For this review, take the finished solid that the model builds, in its own axes (mm). Give positions to 0.01 mm unless a question says otherwise; leave off trailing zeros. Order: outer loops, then holes, each group sorted by start corner. A loop starts at its lowest first (then second) coordinate and runs counter-clockwise, first axis right, second up.
from build123d import *

# Parameters (mm, degrees)
ESQUISSE1_W             = 30
ESQUISSE1_H             = 51
ESQUISSE1_W_2           = 20
ESQUISSE1_H_2           = 41
BOSS_EXTRU_1_DEPTH      = 5
BOSS_EXTRU_3_DEPTH      = 5
BOSS_EXTRU_4_DEPTH      = 8
ESQUISSE5_W             = 30
ESQUISSE5_H             = 5
BOSS_EXTRU_5_DEPTH      = 2.5
ESQUISSE6_W             = 30
ESQUISSE6_H             = 5
BOSS_EXTRU_6_DEPTH      = 2.5
ESQUISSE7_R             = 1.5
ENL_V_MAT_EXTRU_1_DEPTH = 150.584223767
ESQUISSE8_R             = 2.625
ENL_V_MAT_EXTRU_2_DEPTH = 150.584223767
BOSS_EXTRU_8_DEPTH      = 5
BOSS_EXTRU_9_DEPTH      = 31
BOSS_EXTRU_11_DEPTH     = 5
ESQUISSE16_W            = 17
ESQUISSE16_H            = 10
ESQUISSE16_R            = 1.5
BOSS_EXTRU_12_DEPTH     = 5
CHANFREIN3_SIZE         = 0.25
BOSS_EXTRU_13_DEPTH     = 5
BOSS_EXTRU_14_DEPTH     = 5


with BuildPart() as part:
    # Esquisse1 → Boss.-Extru.1 (new body)
    with BuildSketch(Plane.XY):
        Rectangle(ESQUISSE1_W, ESQUISSE1_H)
        Rectangle(ESQUISSE1_W_2, ESQUISSE1_H_2, mode=Mode.SUBTRACT)
    extrude(amount=BOSS_EXTRU_1_DEPTH)

    # Esquisse3 → Boss.-Extru.3 (add)
    with BuildSketch(Plane(origin=(0, 8, 0), x_dir=(1, 0, 0), z_dir=(0, 1, 0))):
        with BuildLine():
            Line((130.711195077, 0), (15, 0))
            Line((15, 0), (15, -5))
            Line((15, -5), (123.166385806, -5))
            ThreePointArc((123.166385806, -5), (125.435495458, -5.705892931), (126.903730879, -7.574429307))
            Line((126.903730879, -7.574429307), (135, -28.8))
            Line((135, -28.8), (145, -28.8))
            Line((145, -28.8), (134.422141223, -2.507057034))
            ThreePointArc((134.422141223, -2.507057034), (132.950416832, -0.685503668), (130.711195077, 0))
        make_face()
        with BuildLine():
            Line((-123.166385806, -5), (-15, -5))
            Line((-15, -5), (-15, 0))
            Line((-15, 0), (-130.711195077, 0))
            ThreePointArc((-130.711195077, 0), (-132.950416832, -0.685503668), (-134.422141223, -2.507057034))
            Line((-134.422141223, -2.507057034), (-145, -28.8))
            Line((-145, -28.8), (-135, -28.8))
            Line((-135, -28.8), (-126.903730879, -7.574429307))
            ThreePointArc((-126.903730879, -7.574429307), (-125.435495458, -5.705892931), (-123.166385806, -5))
        make_face()
    extrude(amount=-BOSS_EXTRU_3_DEPTH)

    # Esquisse4 → Boss.-Extru.4 (add)
    with BuildSketch(Plane(origin=(0, 8, 0), x_dir=(-1, 0, 0), z_dir=(0, 1, 0))):
        Polygon((145, 28.8), (135, 28.8), (133.09280296, 23.8), (142.98846048, 23.8), align=None)
        Polygon((-142.98846048, 23.8), (-145, 28.8), (-135, 28.8), (-133.09280296, 23.8), align=None)
    extrude(amount=BOSS_EXTRU_4_DEPTH)

    # Esquisse5 → Boss.-Extru.5 (add)
    with BuildSketch(Plane(origin=(0, 25.5, 0), x_dir=(1, 0, 0), z_dir=(0, 1, 0))):
        with Locations((0, -2.5)):
            Rectangle(ESQUISSE5_W, ESQUISSE5_H)
    extrude(amount=BOSS_EXTRU_5_DEPTH)

    # Esquisse6 → Boss.-Extru.6 (add)
    with BuildSketch(Plane.XZ.offset(25.5)):
        with Locations((0, 2.5)):
            Rectangle(ESQUISSE6_W, ESQUISSE6_H)
    extrude(amount=BOSS_EXTRU_6_DEPTH)

    # Esquisse7 → Enlèv. mat.-Extru.1 (cut, through all)
    with BuildSketch(Plane(origin=(0, 0, 23.8), x_dir=(-1, 0, 0), z_dir=(0, 0, -1))):
        with Locations((-140, 10)):
            Circle(ESQUISSE7_R)
        with Locations(Location((140, 10, 0), (0, 0, 180))):
            Circle(ESQUISSE7_R)
    extrude(amount=-ENL_V_MAT_EXTRU_1_DEPTH, mode=Mode.SUBTRACT)

    # Esquisse8 → Enlèv. mat.-Extru.2 (cut, through all)
    with BuildSketch(Plane.XY.offset(5)):
        with Locations((-5, 24.925)):
            Circle(ESQUISSE8_R)
        with Locations((5, 24.925)):
            Circle(ESQUISSE8_R)
        with Locations((-5, -25.425)):
            Circle(ESQUISSE8_R)
        with Locations((5, -25.425)):
            Circle(ESQUISSE8_R)
    extrude(amount=-ENL_V_MAT_EXTRU_2_DEPTH, mode=Mode.SUBTRACT)

    # Esquisse12 → Boss.-Extru.8 (add)
    with BuildSketch(Plane(origin=(0, 8, 0), x_dir=(1, 0, 0), z_dir=(0, 1, 0))):
        Polygon((-129.99826692, -15.687214654), (-63.433313414, -5), (-31.892154123, -5), (-132.055900977, -21.081607615), align=None)
        Polygon((132.055900977, -21.081607615), (129.99826692, -15.687214654), (63.433313414, -5), (31.892154123, -5), align=None)
    extrude(amount=-BOSS_EXTRU_8_DEPTH)

    # Esquisse13 → Boss.-Extru.9 (add, through all)
    with BuildSketch(Plane.XZ.offset(-3)):
        with BuildLine():
            Line((-126.684620904, 7), (-136.229687691, 7))
            Line((-136.229687691, 7), (-134.422141223, 2.507057034))
            ThreePointArc((-134.422141223, 2.507057034), (-132.950416832, 0.685503668), (-130.711195077, 0))
            Line((-130.711195077, 0), (-126.684620904, 0))
            Line((-126.684620904, 0), (-126.684620904, 7))
        make_face()
        with BuildLine():
            ThreePointArc((134.422141223, 2.507057034), (132.950416832, 0.685503668), (130.711195077, 0))
            Line((130.711195077, 0), (126.684620904, 0))
            Line((126.684620904, 0), (126.684620904, 7))
            Line((126.684620904, 7), (136.229687691, 7))
            Line((136.229687691, 7), (134.422141223, 2.507057034))
        make_face()
    extrude(amount=BOSS_EXTRU_9_DEPTH)

    # Esquisse15 → Boss.-Extru.11 (add)
    with BuildSketch(Plane(origin=(-114.828371074, 0, -46.196361295), x_dir=(-0.3732357415464263, 0, 0.9277365365405684), z_dir=(-0.9277365365405683, 0, -0.37323574154642625))):
        Polygon((56.042576064, -14.320508076), (66.042576064, 3), (69.506677679, 3), (56.409919429, -19.684250702), align=None)
    boss_extru_11 = extrude(amount=-BOSS_EXTRU_11_DEPTH)

    # Symétrie3: Boss.-Extru.11 across plane
    add(boss_extru_11.mirror(Plane(origin=(0, 0, 0), x_dir=(0, 0, 1), z_dir=(1, 0, 0))))

    # Esquisse16 → Boss.-Extru.12 (add)
    # profile 1 of 2: a face of its own
    with BuildSketch(Plane.XZ.offset(28)):
        with Locations((131.457154298, 3.5)):
            Rectangle(ESQUISSE16_W, ESQUISSE16_H)
        with Locations(Location((124.957154298, 3.5, 0), (0, 0, 270))):
            Circle(ESQUISSE16_R, mode=Mode.SUBTRACT)
        with Locations(Location((137.957154298, 3.5, 0), (0, 0, 90))):
            Circle(ESQUISSE16_R, mode=Mode.SUBTRACT)
    # profile 2 of 2: a face of its own
    with BuildSketch(Plane.XZ.offset(28)):
        with Locations((-131.457154298, 3.5)):
            Rectangle(ESQUISSE16_W, ESQUISSE16_H)
        with Locations(Location((-137.957154298, 3.5, 0), (0, 0, 270))):
            Circle(ESQUISSE16_R, mode=Mode.SUBTRACT)
        with Locations(Location((-124.957154298, 3.5, 0), (0, 0, 90))):
            Circle(ESQUISSE16_R, mode=Mode.SUBTRACT)
    extrude(amount=BOSS_EXTRU_12_DEPTH)

    # Chanfrein3
    chanfrein3_edges = [part.edges().sort_by_distance(p)[0] for p in [
        (139.957154298, -28, 3.5),
        (131.457154298, -28, 8.5),
        (122.957154298, -28, 3.5),
        (131.457154298, -28, -1.5),
        (-122.957154298, -28, 3.5),
        (-131.457154298, -28, 8.5),
        (-139.957154298, -28, 3.5),
        (-131.457154298, -28, -1.5),
    ]]
    chamfer(chanfrein3_edges, length=CHANFREIN3_SIZE)

    # Esquisse17 → Boss.-Extru.13 (add)
    with BuildSketch(Plane(origin=(-20.455095506, 3.753380181, 50.844378892), x_dir=(-0.9280869704105542, -0.02741363174056612, -0.37135302361627764), z_dir=(0.3723634989551998, -0.06832633838021179, -0.9255684394626872))):
        Polygon((119.373285615, -20.220046325), (122.060546569, -20.146178288), (121.000071898, -14.796991142), (119.225556278, -14.845769429), align=None)
    extrude(amount=BOSS_EXTRU_13_DEPTH)

    # Esquisse18 → Boss.-Extru.14 (add)
    with BuildSketch(Plane(origin=(20.455095506, 3.753380181, 50.844378892), x_dir=(-0.9280869704105542, 0.02741363174056612, 0.37135302361627764), z_dir=(-0.3723634989551998, -0.06832633838021179, -0.9255684394626872))):
        Polygon((-119.225556278, -14.845769429), (-121.000071898, -14.796991142), (-122.060546569, -20.146178288), (-119.373285615, -20.220046325), align=None)
    extrude(amount=BOSS_EXTRU_14_DEPTH)


solid = part.part
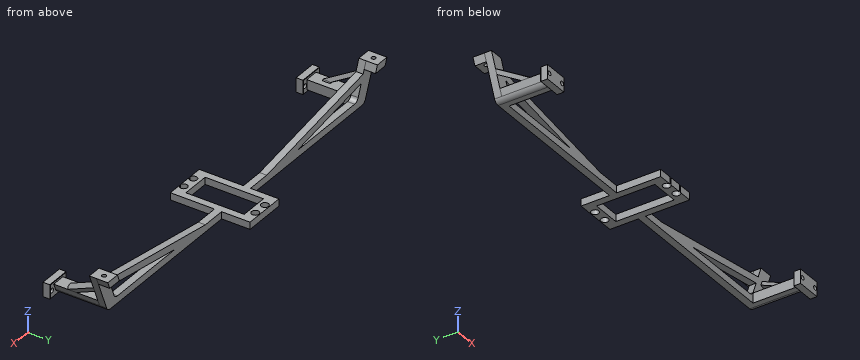
1) We need section A-A on y = -6. Give the boundary of the cut face in (x, z).
Answer sheet:
outline: (-138.83, 13.47) - (-137.54, 10.25) - (-132.9, 12.12) - (-134.19, 15.33) - close; (-136.23, 7) - (-134.42, 2.51) arc R4 ccw to (-130.71, 0) - (-126.68, 0) - (-126.68, 7) - close; (-15, 0) - (-10, 0) - (-10, 5) - (-15, 5) - close; (10, 0) - (15, 0) - (15, 5) - (10, 5) - close; (126.68, 0) - (130.71, 0) arc R4 ccw to (134.42, 2.51) - (136.23, 7) - (126.68, 7) - close; (132.9, 12.12) - (137.54, 10.25) - (138.83, 13.47) - (134.19, 15.33) - close
2) To check wall thickness, follow line 1 (X direction, y = -31.8, z = 3.5); line 2 (Y direction, x = -5, z = 2.95); line 3 (X direction, y = 9.5, z = 25.5). State the ranges of each line that lie inside material, in increasing order.
Answer sheet:
line 1: x = -139.96 to -139.46, -136.46 to -126.46, -123.46 to -122.96, 122.96 to 123.46, 126.46 to 136.46, 139.46 to 139.96
line 2: y = -22.8 to -20.5, 20.5 to 22.3, 27.55 to 28
line 3: x = -143.67 to -141.41, -138.59 to -133.74, 133.74 to 138.59, 141.41 to 143.67
3) We need section B-B on x = -94. Give the boundary of the cut face in (y, z), then the cut area to 3 significant figures.
Answer sheet:
outline: (3, 0) - (8, 0) - (8, 5) - (3, 5) - close; (3, 9.91) - (8, 9.91) - (8, 14.97) - (3, 14.97) - close
area: 50.3 mm2
4) Clearance check with flat-ended pins moving along their axes: pin 1 (2.5 mm diameter, centred on x = 137, y = 12, fed in from -Z); pin 2 (5 mm diameter, centred on x = -135, y = -29.5, fed in from +Z); pin 3 (5.5 mm diameter, centred on y = 14.5, z = 3.5, fed in from -X). State where each tip first meets the part, or that it passes through.
Answer sheet:
pin 1: stops at z = 23.8
pin 2: stops at z = 8.5
pin 3: stops at x = -15
